The listing builds one solid part. Answer for the finished solid, in the listing's coordinates (mm). A direction names the side the tool comes from. Give positions to 0.01 mm unless a question says otherwise; leave off trailing zeros. Write each loop counter-clockwise with the first axis right and the second up, starting at its lowest first coordinate (ties: lowest second). Pieces come first, ordered by that corner, then holes. Notation, with made-up numbers: (-18, 14.5) - (3, 14.5) arc R18 cw to (3, 21.5) - close; hole circle Ø1 at (55.5, -5.5). An arc over 180 degrees is marked (long way). Return JSON: item names as keys, results as strings.
from build123d import *

# Parameters (mm, degrees)
BOSS_EXTRUDE1_DEPTH = 592.455
CUT_EXTRUDE1_DEPTH  = 482.6
BOSS_EXTRUDE2_DEPTH = 6.35
BOSS_EXTRUDE3_DEPTH = 6.35
SKETCH5_R           = 158.75
BOSS_EXTRUDE4_DEPTH = 12.7
SKETCH6_R           = 158.75
SKETCH6_R_2         = 152.4
BOSS_EXTRUDE5_DEPTH = 88.9


with BuildPart() as part:
    # Sketch1 → Boss-Extrude1 (new body, symmetric)
    with BuildSketch(Plane(origin=(0, 0, 0), x_dir=(0, 0, -1), z_dir=(1, 0, 0))):
        with BuildLine():
            Line((128.652963539, -19.049996224), (-128.652963539, -19.049996224))
            ThreePointArc((-128.652963539, -19.049996224), (-131.083003335, -19.533361193), (-133.1430916, -20.909868164))
            Line((-133.1430916, -20.909868164), (-239.440128061, -127.206904624))
            ThreePointArc((-239.440128061, -127.206904624), (-240.816635031, -129.266992889), (-241.3, -131.697032685))
            Line((-241.3, -131.697032685), (-241.3, -253.999996224))
            Line((-241.3, -253.999996224), (-234.95, -253.999996224))
            Line((-234.95, -253.999996224), (-234.95, -134.327288806))
            ThreePointArc((-234.95, -134.327288806), (-234.466635031, -131.89724901), (-233.090128061, -129.837160745))
            Line((-233.090128061, -129.837160745), (-130.512835479, -27.259868164))
            ThreePointArc((-130.512835479, -27.259868164), (-128.452747214, -25.883361193), (-126.022707418, -25.399996224))
            Line((-126.022707418, -25.399996224), (126.022707418, -25.399996224))
            ThreePointArc((126.022707418, -25.399996224), (128.452747214, -25.883361193), (130.512835479, -27.259868164))
            Line((130.512835479, -27.259868164), (233.090128061, -129.837160745))
            ThreePointArc((233.090128061, -129.837160745), (234.466635031, -131.89724901), (234.95, -134.327288806))
            Line((234.95, -134.327288806), (234.95, -253.999996224))
            Line((234.95, -253.999996224), (241.3, -253.999996224))
            Line((241.3, -253.999996224), (241.3, -131.697032685))
            ThreePointArc((241.3, -131.697032685), (240.816635031, -129.266992889), (239.440128061, -127.206904624))
            Line((239.440128061, -127.206904624), (133.1430916, -20.909868164))
            ThreePointArc((133.1430916, -20.909868164), (131.083003335, -19.533361193), (128.652963539, -19.049996224))
        make_face()
    extrude(amount=BOSS_EXTRUDE1_DEPTH, both=True)

    # Sketch2 → Cut-Extrude1 (cut)
    with BuildSketch(Plane(origin=(0, 0, -241.3), x_dir=(-1, 0, 0), z_dir=(0, 0, -1))):
        Polygon((-592.455, -253.999996224), (-378.079, -253.999996224), (-592.455, -25.399996224), align=None)
        Polygon((-535.401348451, -27.939996224), (-467.080186427, -102.818047021), (-482.955186427, -120.216595599), (-567.151348451, -27.939996224), align=None)
        Polygon((-398.759024402, -27.939996224), (-419.455186427, -50.622401287), (-440.151348451, -27.939996224), align=None)
        Polygon((-503.651348451, -27.939996224), (-451.205186427, -85.419498443), (-435.330186427, -68.020949865), (-471.901348451, -27.939996224), align=None)
        Polygon((398.759024402, -27.939996224), (440.151348451, -27.939996224), (419.455186427, -50.622401287), align=None)
        Polygon((471.901348451, -27.939996224), (503.651348451, -27.939996224), (451.205186427, -85.419498443), (435.330186427, -68.020949865), align=None)
        Polygon((535.401348451, -27.939996224), (567.151348451, -27.939996224), (482.955186427, -120.216595599), (467.080186427, -102.818047021), align=None)
        Polygon((592.455, -25.399996224), (592.455, -253.999996224), (378.079, -253.999996224), align=None)
    extrude(amount=-CUT_EXTRUDE1_DEPTH, mode=Mode.SUBTRACT)

    # Sketch3 → Boss-Extrude2 (add)
    with BuildSketch(Plane(origin=(0, 0, -241.3), x_dir=(-1, 0, 0), z_dir=(0, 0, -1))):
        Polygon((-372.124111111, -260.349996224), (372.124111111, -260.349996224), (378.079, -253.999996224), (-378.079, -253.999996224), align=None)
    extrude(amount=-BOSS_EXTRUDE2_DEPTH)

    # Sketch4 → Boss-Extrude3 (add)
    with BuildSketch(Plane.XY.offset(241.3)):
        Polygon((-372.124111111, -260.349996224), (372.124111111, -260.349996224), (378.079, -253.999996224), (-378.079, -253.999996224), align=None)
    extrude(amount=-BOSS_EXTRUDE3_DEPTH)

    # Sketch5 → Boss-Extrude4 (add)
    with BuildSketch(Plane(origin=(0, -19.049996224, 0), x_dir=(1, 0, 0), z_dir=(0, 1, 0))):
        Circle(SKETCH5_R)
    extrude(amount=BOSS_EXTRUDE4_DEPTH)

    # Sketch6 → Boss-Extrude5 (add)
    with BuildSketch(Plane(origin=(0, -6.349996224, 0), x_dir=(1, 0, 0), z_dir=(0, 1, 0))):
        Circle(SKETCH6_R)
        Circle(SKETCH6_R_2, mode=Mode.SUBTRACT)
    extrude(amount=BOSS_EXTRUDE5_DEPTH)


solid = part.part
Item 1: Flat-ended cylindrical pins translate along their axes: P1, Ø6, axis at x = 299.5, y = -18, coming from the -Z side; P2, Ø2.5, axis at x = -545.5, z = 136.5, coming from the -Y side; P3, Ø1, axis at y = 32.5, z = 50, coming from the +X side. Find the tip coordinate at first contact, or state that the pin passes through.
Answer below:
{"P1": "stops at z = -133.23", "P2": "stops at y = -27.94", "P3": "stops at x = 150.84"}
Item 2: A cutting plane is placed at D-D on x = 134. Determine the outline of the cut face in (y, z).
Answer below:
{"outline": "(-260.35, -241.3) - (-131.7, -241.3) arc R6.35 ccw to (-127.21, -239.44) - (-20.91, -133.14) arc R6.35 ccw to (-19.05, -128.65) - (-19.05, -85.12) - (82.55, -85.12) - (82.55, -72.59) - (-6.35, -72.59) - (-6.35, 72.59) - (82.55, 72.59) - (82.55, 85.12) - (-19.05, 85.12) - (-19.05, 128.65) arc R6.35 ccw to (-20.91, 133.14) - (-127.21, 239.44) arc R6.35 ccw to (-131.7, 241.3) - (-260.35, 241.3) - (-260.35, 234.95) - (-134.33, 234.95) arc R6.35 cw to (-129.84, 233.09) - (-27.26, 130.51) arc R6.35 cw to (-25.4, 126.02) - (-25.4, -126.02) arc R6.35 cw to (-27.26, -130.51) - (-129.84, -233.09) arc R6.35 cw to (-134.33, -234.95) - (-260.35, -234.95) - close"}
Item 3: A cutting plane is placed at C-C on x = -287.5. Determine the outline of the cut face in (y, z).
Answer below:
{"outline": "(-260.35, -241.3) - (-131.7, -241.3) arc R6.35 ccw to (-127.21, -239.44) - (-20.91, -133.14) arc R6.35 ccw to (-19.05, -128.65) - (-19.05, 128.65) arc R6.35 ccw to (-20.91, 133.14) - (-127.21, 239.44) arc R6.35 ccw to (-131.7, 241.3) - (-260.35, 241.3) - (-260.35, 234.95) - (-134.33, 234.95) arc R6.35 cw to (-129.84, 233.09) - (-27.26, 130.51) arc R6.35 cw to (-25.4, 126.02) - (-25.4, -126.02) arc R6.35 cw to (-27.26, -130.51) - (-129.84, -233.09) arc R6.35 cw to (-134.33, -234.95) - (-260.35, -234.95) - close"}
Item 4: A cutting plane is placed at A-A on z = 0. Determine the outline of the cut face in (x, y) (3 decimals).
Answer below:
{"outline": "(-592.455, -25.4) - (592.455, -25.4) - (592.455, -19.05) - (158.75, -19.05) - (158.75, 82.55) - (152.4, 82.55) - (152.4, -6.35) - (-152.4, -6.35) - (-152.4, 82.55) - (-158.75, 82.55) - (-158.75, -19.05) - (-592.455, -19.05) - close"}
Item 5: The mould has two halves that part along X. Classify faces 4 (the face through (7, -196, -234.95)), 5 (the face through (-429.85, -39.23, -145.93)): +X half, -X half, draft (parallel to the pull), parting line (faces both ways), or undercut.
Answer below:
{"face 4": "draft", "face 5": "undercut"}
Item 6: For faces 1 (the face through (7, -195, -241.3)), 2 (the face through (-2, -6.35, -2)), 3 (the face through (8.27, -79.267, 182.52)), determine the directions among +Z, -Z, +X, -X, +Y, -Y from which every point of the face is accessible in a straight line to the end or side of a thin tool.
Answer below:
{"face 1": "-Z, +X, -X, +Y, -Y", "face 2": "+Y", "face 3": "+X, -X, -Y"}
Item 7: Consider L1, parallel to Z at x = 0, y = 12; L2, parallel to Z at x = -378, y = -193.5. Determine where each line is inside the solid, lowest interval first.
Answer below:
{"L1": "z = -158.75 to -152.4, 152.4 to 158.75", "L2": "z = -241.3 to -234.95, 234.95 to 241.3"}
Item 8: A cutting plane is placed at B-B on y = -204. Determine the outline of the cut face in (x, z), then the cut area to 3 significant figures.
Answer below:
{"outline": "(-424.97, -241.3) - (424.97, -241.3) - (424.97, -234.95) - (-424.97, -234.95) - close; (-424.97, 234.95) - (424.97, 234.95) - (424.97, 241.3) - (-424.97, 241.3) - close", "area": "10,800 mm²"}
